from build123d import *

# Parameters (mm, degrees)
BOSS_EXTRUDE1_DEPTH           = 1.6
M3_CLEARANCE_HOLE1_AT_2_COUNT = 2
M3_CLEARANCE_HOLE1_AT_2_PITCH = 33
FILLET1_R                     = 2


with BuildPart() as part:
    # Sketch1 → Boss-Extrude1 (new body)
    with BuildSketch(Plane.XY):
        with BuildLine():
            Line((8, 19), (-8, 19))
            Line((-8, 19), (-19, 38.052558883))
            Line((-19, 38.052558883), (-19, 47.073195958))
            Line((-19, 47.073195958), (-7.75, 47.073195958))
            ThreePointArc((-7.75, 47.073195958), (-6.578427125, 44.244768833), (-3.75, 43.073195958))
            Line((-3.75, 43.073195958), (3.75, 43.073195958))
            ThreePointArc((3.75, 43.073195958), (6.578427125, 44.244768833), (7.75, 47.073195958))
            Line((7.75, 47.073195958), (19, 47.073195958))
            Line((19, 47.073195958), (19, 38.052558883))
            Line((19, 38.052558883), (8, 19))
        make_face()
    extrude(amount=BOSS_EXTRUDE1_DEPTH)

    # Sketch3 → M3 Clearance Hole1 (revolve, cut)
    with BuildSketch(Plane(origin=(16.5, 44.573195958, 1.6), x_dir=(0, -1, 0), z_dir=(1, 0, 0))):
        Polygon((0, 0), (0, 1.6), (1.6, 1.6), (1.6, 0.025), (1.625, 0), align=None)
    m3_clearance_hole1 = revolve(axis=Axis((16.5, 44.573195958, 7.95), (0, 0, -1)), mode=Mode.SUBTRACT)

    # M3 Clearance Hole1 at 2: M3 Clearance Hole1 ×2
    with Locations(*[(-i * M3_CLEARANCE_HOLE1_AT_2_PITCH, 0, 0) for i in range(1, M3_CLEARANCE_HOLE1_AT_2_COUNT)]):
        add(m3_clearance_hole1, mode=Mode.SUBTRACT)

    # Fillet1
    fillet1_edges = [part.edges().sort_by_distance(p)[0] for p in [
        (-19, 47.073195958, 0.8),
        (-7.75, 47.073195958, 0.8),
        (7.75, 47.073195958, 0.8),
        (19, 47.073195958, 0.8),
        (19, 38.052558883, 0.8),
        (-19, 38.052558883, 0.8),
    ]]
    fillet(fillet1_edges, radius=FILLET1_R)


solid = part.part
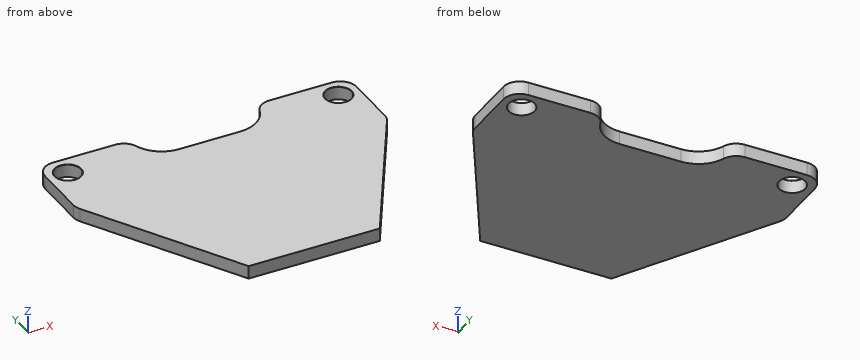
Can you work these out from the model? Positions are in its coordinate system, mm. Coordinates: 2 decimals unless noted, no trailing zeros. Loops run counter-clockwise (first coordinate to the right, second up) from the corner with the lowest first, then second, coordinate; pieces in that order, holes last. Notation, with made-up numbers: (-39, 4.5) - (9, 4.5) arc R4 cw to (9, 9.5) - close; hole circle Ø7 at (72, 29.25). An arc over 180 degrees is marked (long way). Put each result on its own line as item: value. Start each with the question number.
Item 1: Suppose I cut it at C-C (x = 8.5). Please give me the cut outline in (y, z).
Item 2: For pin 1 (2.5 mm diameter, centred on x = -16.5, y = 44.57, fed in from -Z); pin 2 (0.8 mm diameter, centred on x = -1, z = 1, fed in from +Y), each with a flat end and sliding along its axis, tell me the tip position at first contact or that it passes through.
Item 3: Suppose I cut it at A-A (z = 1.2). Please give me the cut outline in (x, y).
Item 4: Suppose I cut it at D-D (y = 23.25). Please give me the cut outline in (x, z).
Item 5: Suppose I cut it at B-B (x = 16.5). Please give me the cut outline in (y, z) (3 decimals), and give its area (3 significant figures).
Item 6: If I drill on line 1 along Y through (x, z) = (16.5, 0.6); line 2 along X through (y, z) = (45, 0.4); line 3 along X through (y, z) = (36, 0.2), over which ranges is the centre line in solid material (lowest first)?
Here are the results:
1. outline: (19.87, 0) - (46.86, 0) - (46.86, 1.6) - (19.87, 1.6) - close
2. pin 1: through
2. pin 2: y = 43.07
3. outline: (-19, 38.59) arc R2 ccw to (-18.73, 37.59) - (-8, 19) - (8, 19) - (18.73, 37.59) arc R2 ccw to (19, 38.59) - (19, 45.07) arc R2 ccw to (17, 47.07) - (9.41, 47.07) arc R2 ccw to (7.52, 45.74) arc R4 cw to (3.75, 43.07) - (-3.75, 43.07) arc R4 cw to (-7.52, 45.74) arc R2 ccw to (-9.41, 47.07) - (-17, 47.07) arc R2 ccw to (-19, 45.07) - close; hole circle Ø3.2 at (-16.5, 44.57); hole circle Ø3.2 at (16.5, 44.57)
4. outline: (-10.45, 0) - (10.45, 0) - (10.45, 1.6) - (-10.45, 1.6) - close
5. outline: (33.722, 0) - (42.973, 0) - (42.973, 1.575) - (42.948, 1.6) - (33.722, 1.6) - close; (46.173, 0) - (47.073, 0) - (47.073, 1.6) - (46.198, 1.6) - (46.173, 1.575) - close
5. area: 16.2 mm²
6. line 1: 33.72 to 42.97, 46.17 to 47.07
6. line 2: -19 to -18.04, -14.96 to -7.17, 7.17 to 14.96, 18.04 to 19
6. line 3: -17.81 to 17.81
